Check sheet for the modelled part. Datum: model origin and axes. Units: mm. A direction names the side the tool comes from. Coordinates: 2 decimals unless noted, no trailing zeros. Write each loop counter-clockwise with the first axis right and the second up, starting at its lowest first coordinate (ties: lowest second). Pieces come first, ordered by that corner, then holes. Notation, with made-up numbers: M 35.5,-25.75 L 60.5,-25.75 A26 cw 60.5,-7.75 Z; hole C -4,-11.75 d2. An arc over 180 degrees is marked long. Answer as CSV lines item,"result". Start each with the question number.
Q1. Thickness scan on line 1 along Z through (x, y) = (23.57, -14.5) (3 decimals); line 2 along Z through (x, y) = (40, -7.75) (3 decimals); line 3 along Z through (x, y) = (44, -12) (3 decimals). Record the ranges inside material, lowest first. Write a range as from..to.
Q2. Mould release check, pull along X, two halves, no side actions. Record for faces 1 (the cylindrical face through (-40.461, -5.07, 8.926)), 2 (the flat face through (50, -9.5, -0.4)), 3 (the flat face through (34, -25, -24)), 4 (the flat face through (-1, -10, 0)): pulls with the +X half, pulls with the -X half, needs draft (parallel to the pull), parting line crosses it, or undercut.
Q3. Sectioned sample at D-D, the plane y = -6. Count the separate pieces of the cut face and the enclosed holes in it, then the cut area to 3 significant figures.
Q4. Sectioned sample at B-B, the plane z = -11. Record the cut outline in (x, y) (3 decimals), then the cut area to 3 significant figures.
Q5. Depth check by flat-ended pin: pin 1 Ø7 at (x, z) = (40, 11) entering from -Y. Enter the tip coordinate at first touch or a pass-through.
Q6. Sectioned sample at C-C, the plane x = 40. Record the cut outline in (y, z) (3 decimals), then the cut area to 3 significant figures.
Q7. Sectioned sample at A-A, the plane y = -23.5. Record the cut outline in (x, z) (3 decimals), then the cut area to 3 significant figures.
Q8. Access from +Z, -Z, +X, -X, +Y, -Y to the whole of each face (thin tool, end or side, straight path). Record for faces 5 (the flat face through (-35, -18, 18.895)), 6 (the cylindrical face through (-40.461, -5.07, -13.074)), 7 (the flat face through (-18.895, -18, 24)).
from build123d import *

# Parameters (mm, degrees)
F0_W     = 100
F0_H     = 60
F1_DEPTH = 25
F3_W     = 100
F3_H     = 37.79
F4_DEPTH = 15
F2_R     = 2.675
F5_DEPTH = 25.001
F6_R     = 2.125
F7_DEPTH = 10.001
F8_W     = 37.79
F8_H     = 60
F9_DEPTH = 15


with BuildPart() as f1:
    # F0 (on Front) → F1 (new body)
    with BuildSketch(Plane.XZ):
        Rectangle(F0_W, F0_H)
    extrude(amount=F1_DEPTH)

    # F3 (on face) → F4 (cut)
    with BuildSketch(Plane.XZ.offset(25)):
        Rectangle(F3_W, F3_H)
    extrude(amount=-F4_DEPTH, mode=Mode.SUBTRACT)

    # F2 (on face) → F5 (cut, through all)
    with BuildSketch(Plane.XZ.offset(25)):
        with Locations((-23.57, 23.57)):
            Circle(F2_R)
        with Locations((23.57, 23.57)):
            Circle(F2_R)
        with Locations((-23.57, -23.57)):
            Circle(F2_R)
        with Locations((23.57, -23.57)):
            Circle(F2_R)
    extrude(amount=-F5_DEPTH, mode=Mode.SUBTRACT)

    # F6 (on face) → F7 (cut, through all)
    with BuildSketch(Plane.XZ.offset(10)):
        with Locations((-40, 11)):
            Circle(F6_R)
        with Locations((-40, -11)):
            Circle(F6_R)
        with Locations((40, 11)):
            Circle(F6_R)
        with Locations((40, -11)):
            Circle(F6_R)
    extrude(amount=-F7_DEPTH, mode=Mode.SUBTRACT)

    # F8 (on face) → F9 (cut)
    with BuildSketch(Plane.XZ.offset(25)):
        Rectangle(F8_W, F8_H)
    extrude(amount=-F9_DEPTH, mode=Mode.SUBTRACT)


solid = f1.part
Output:
1,line 1,"z = -30..-26.245, -20.895..-18.895, 18.895..20.895, 26.245..30"
1,line 2,"z = -30..-13.125, -8.875..8.875, 13.125..30"
1,line 3,"z = -30..-18.895, 18.895..30"
2,face 1,"undercut"
2,face 2,"pulls with the +X half"
2,face 3,"needs draft"
2,face 4,"undercut"
3,separate pieces,"1"
3,enclosed holes,"8"
3,area,"5,850 mm^2"
4,outline,"M -50,-10 L -42.125,-10 L -42.125,0 L -50,0 Z; M -37.875,-10 L 37.875,-10 L 37.875,0 L -37.875,0 Z; M 42.125,-10 L 50,-10 L 50,0 L 42.125,0 Z"
4,area,"915 mm^2"
5,pin 1,"stops at y = -10"
6,outline,"M -25,-30 L 0,-30 L 0,-13.125 L -10,-13.125 L -10,-18.895 L -25,-18.895 Z; M -25,18.895 L -10,18.895 L -10,13.125 L 0,13.125 L 0,30 L -25,30 Z; M -10,-8.875 L 0,-8.875 L 0,8.875 L -10,8.875 Z"
6,area,"848 mm^2"
7,outline,"M -50,-30 L -18.895,-30 L -18.895,-18.895 L -50,-18.895 Z; M -50,18.895 L -18.895,18.895 L -18.895,30 L -50,30 Z; M 18.895,-30 L 50,-30 L 50,-18.895 L 18.895,-18.895 Z; M 18.895,18.895 L 50,18.895 L 50,30 L 18.895,30 Z; hole C -23.57,-23.57 d5.35; hole C -23.57,23.57 d5.35; hole C 23.57,-23.57 d5.35; hole C 23.57,23.57 d5.35"
7,area,"1,290 mm^2"
8,face 5,"+X, -X, -Y"
8,face 6,"+Y, -Y"
8,face 7,"+Z, -Z, -Y"
